from build123d import *

# Parameters (mm, degrees)
F0_W     = 4.1275
F0_H     = 46.6725
F0_H_2   = 4.1275
F0_W_2   = 46.6725
F1_DEPTH = 127
F4_D     = 6.35
F5_D     = 6.35
F6_D     = 6.35
F7_D     = 6.35


with BuildPart() as f1:
    # F0 (on Front) → F1 (new body)
    with BuildSketch(Plane.XZ):
        with Locations((-64.07842, -10.049134)):
            Rectangle(F0_W, F0_H)
        with Locations((-64.07842, -35.449134)):
            Rectangle(F0_W, F0_H_2)
        with Locations((-89.47842, -35.449134)):
            Rectangle(F0_W_2, F0_H_2)
    extrude(amount=F1_DEPTH)

    # F4 (through all)
    with Locations(Plane.YZ.offset(-62.01467)):
        with Locations((-101.6, -12.112884)):
            Hole(F4_D / 2)

    # F5 (through all)
    with Locations(Plane(origin=(0, 0, -37.512884), x_dir=(1, 0, 0), z_dir=(0, 0, -1))):
        with Locations((-87.41467, 101.6)):
            Hole(F5_D / 2)

    # F6 (through all)
    with Locations(Plane.YZ.offset(-62.01467)):
        with Locations((-25.4, -12.112884)):
            Hole(F6_D / 2)

    # F7 (through all)
    with Locations(Plane(origin=(0, 0, -37.512884), x_dir=(1, 0, 0), z_dir=(0, 0, -1))):
        with Locations((-87.41467, 25.4)):
            Hole(F7_D / 2)


solid = f1.part
Could you check a few things on this model? Use its own coordinates, in mm. A direction names the side the tool comes from. Give positions to 0.01 mm unless a question says otherwise; leave off trailing zeros. Write each loop counter-clockwise with the first axis right and the second up, starting at its lowest first coordinate (ties: lowest second). Pieces come first, ordered by that corner, then holes. Notation, with made-up numbers: (34.25, 0.25) -> (81.25, 0.25) arc R21 cw to (81.25, 29.25) -> close; hole circle Ø2 at (-9, 1). An arc over 180 degrees is marked (long way). Write each question's results on one line, items separated by ' | '. Start each with the question number.
Q1. Suppose I cut it at A-A, the plane y = -101.6. List the corners of the cut face in (x, z) for me.
Q2. We'd pull the mould along Y, two halves only. Please class faces 3 (the face through (-90.443, -102.554, -35.42)), 4 (the face through (-62.015, -63, -12)), 5 (the face through (-76, -127, -35)): +Y half, -Y half, draft (parallel to the pull), parting line (faces both ways), or undercut.
Q3. Suppose I cut it at C-C, the plane z = -27.5. List the corners of the cut face in (x, y) for me.
Q4. Suppose I cut it at D-D, the plane x = -109.5. List the corners of the cut face in (y, z) for me.
Q5. Suppose I cut it at B-B, the plane y = -69.5. List the corners of the cut face in (x, z) for me.
Q6. Which directions (+Z, -Z, +X, -X, +Y, -Y) give clear straight access to the entire face, cutting with the end or side of a thin tool? Please do faces 1 (the face through (-90, -63, -33.385)), 2 (the face through (-112.815, -63, -35)).
Q7. I'm going to push flat-ended pins straight in: pin 1 Ø8.5 at (y, z) = (-101.6, -12.11) entering from -X; pin 2 Ø8 at (x, z) = (-73.5, -14) entering from +Y; pin 3 Ø3 at (x, y) = (-100, -110.5) entering from +Z. Where does each tip first touch, or does it pass through?
Q8. I need wall thicknesses on probe 1 along Z at (x, y) = (-63.4, -25.4); probe 2 along Y at (x, z) = (-65.5, -13); probe 3 along X at (y, z) = (-25.4, -35.35). Which ranges of each line are inside material? Lowest first, please.
Outcome:
1) outline: (-112.81, -37.51) -> (-90.59, -37.51) -> (-90.59, -33.39) -> (-112.81, -33.39) -> close; (-84.24, -37.51) -> (-62.01, -37.51) -> (-62.01, -15.29) -> (-66.14, -15.29) -> (-66.14, -33.39) -> (-84.24, -33.39) -> close; (-66.14, -8.94) -> (-62.01, -8.94) -> (-62.01, 13.29) -> (-66.14, 13.29) -> close
2) face 3: undercut | face 4: draft | face 5: -Y half
3) outline: (-66.14, -127) -> (-62.01, -127) -> (-62.01, 0) -> (-66.14, 0) -> close
4) outline: (-127, -37.51) -> (0, -37.51) -> (0, -33.39) -> (-127, -33.39) -> close
5) outline: (-112.81, -37.51) -> (-62.01, -37.51) -> (-62.01, 13.29) -> (-66.14, 13.29) -> (-66.14, -33.39) -> (-112.81, -33.39) -> close
6) face 1: +Z, -X, +Y, -Y | face 2: +Z, -Z, -X, +Y, -Y
7) pin 1: x = -66.14 | pin 2: through | pin 3: z = -33.39
8) probe 1: -37.51 to -15.29, -8.94 to 13.29 | probe 2: -127 to -104.65, -98.55 to -28.45, -22.35 to 0 | probe 3: -112.81 to -90.59, -84.24 to -62.01
